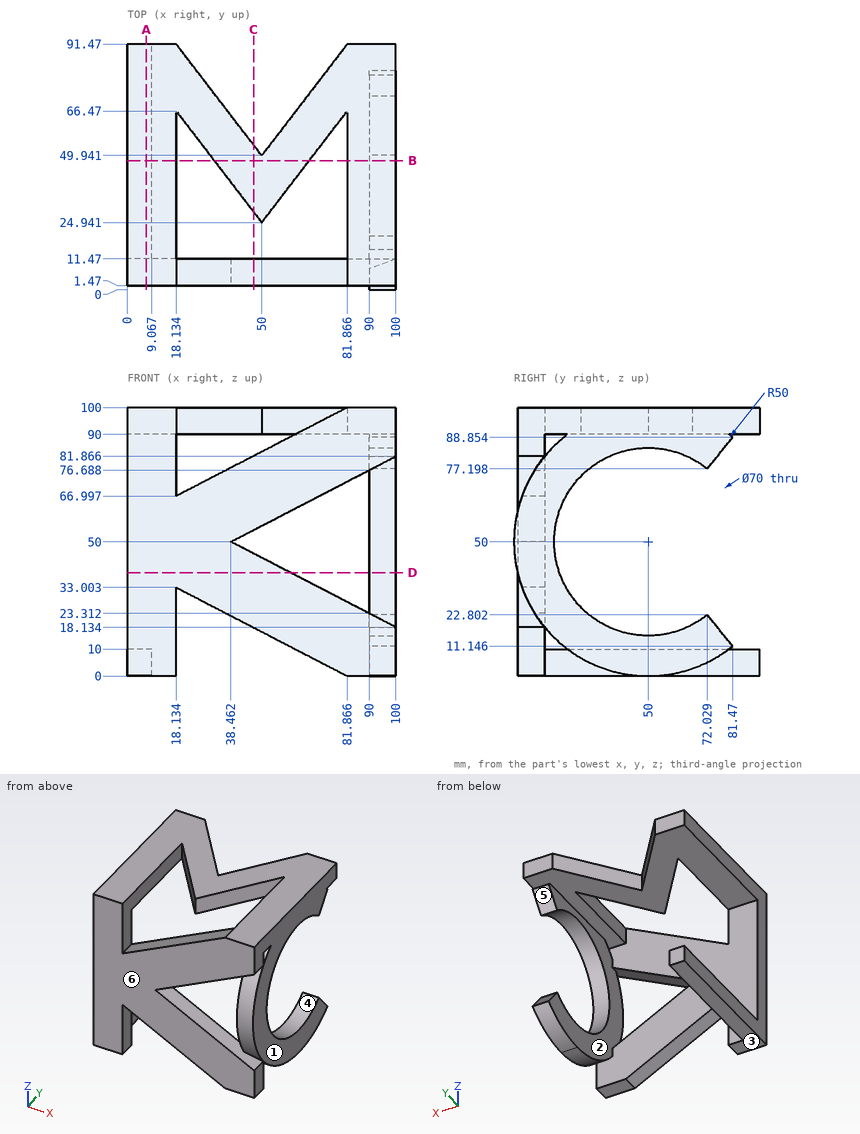
Job drawing, mm, ordinate dimensions from the low corner. One solid piece. A direction names the side the tool comes from. Coordinates: 2 decimals unless noted, no trailing zeros. Order: outer loops, then holes, each group sorted by start corner. A loop starts at its lowest first (then second) coordinate and runs counter-clockwise, first axis right, second up. Notation, with made-up numbers: (74.5, 70.5) - (120.5, 70.5) arc R29 ccw to (120.5, 93.5) - close; hole circle Ø10 at (-8, 16). An arc over 180 degrees is marked (long way). Return JSON: item names as keys, results as strings. Group by question number.
1) Probe line 1 (Z direction, x = 96, y = 50); line 2 (X direction, y = 37.5, z = 91) (1 decimal); line 3 (Y direction, x = 92, z = 50). List the from-to ranges inside material, lowest first. Write a range as from..to.
2) Saw through at B-B, the plane y = 48. Write the cut outline in (x, z), plus the area to 3 significant figures.
3) Saw through at D-D, the plane z = 38.5. Write the cut outline in (x, y), plus the area to 3 significant figures.
4) Flat gauge pins, fed straight in: P1, Ø4, axis at y = 57, z = 86, coming from the -X side; P2, Ø1, axis at x = 25, z = 45, coming from the -Y side; P3, Ø6, axis at x = 69, z = 32, coming from the +Y side. Where does each tip first touch, or does it go through?
5) Mould opens along Y. For the marked faces 3, 4, 5 and 6 say: released by +Y, released by -Y, zero draft, split by the parting line, or undercut.
6) Saw through at C-C, the plane x = 47. Write the cut outline in (y, z) (1 decimal).
7) Tool access for the marked faces 1 and 2: list every direction of +Z, -Z, +X, -X, +Y, -Y with a clear straight run to the whole face (end or side of a thin tool).
8) Saw through at A-A, the plane x = 7. Write the cut outline in (y, z).
Values found:
{
 "1": {"line 1": "z = 0..15, 85..100", "line 2": "x = 0..18.1, 40.4..59.6, 81.9..100", "line 3": "y = 0..15"},
 "2": {"outline": "(0, 0) - (9.07, 0) - (9.07, 10) - (0, 10) - close; (0, 90) - (18.13, 90) - (18.13, 100) - (0, 100) - close; (32.31, 90) - (67.69, 90) - (67.69, 100) - (32.31, 100) - close; (81.87, 90) - (90, 90) - (90, 84.94) - (100, 84.94) - (100, 100) - (81.87, 100) - close; (90, 0.04) - (100, 0.04) - (100, 15.06) - (90, 15.06) - close", "area": "1,010 mm²"},
 "3": {"outline": "(0, 1.47) - (60.67, 1.47) - (60.67, 11.47) - (0, 11.47) - close; (90, 1.34) - (100, 1.34) - (100, 16.94) - (90, 16.94) - close", "area": "763 mm²"},
 "4": {"P1": "stops at x = 90", "P2": "stops at y = 1.47", "P3": "stops at y = 11.47"},
 "5": {"face 3": "zero draft", "face 4": "undercut", "face 5": "released by +Y", "face 6": "released by -Y"},
 "6": {"outline": "(1.5, 18.1) - (11.5, 18.1) - (11.5, 45.6) - (1.5, 45.6) - close; (1.5, 54.4) - (11.5, 54.4) - (11.5, 81.9) - (1.5, 81.9) - close; (28.9, 90) - (53.9, 90) - (53.9, 100) - (28.9, 100) - close"},
 "7": {"face 1": "+Z, -Z, +X, +Y, -Y", "face 2": "+Y"},
 "8": {"outline": "(1.47, 0) - (91.47, 0) - (91.47, 10) - (11.47, 10) - (11.47, 90) - (91.47, 90) - (91.47, 100) - (1.47, 100) - close"}
}
